Design review of the part built by this model. Coordinates are the model's own, in mm. Coordinates: 2 decimals unless noted, no trailing zeros. Write each loop counter-clockwise with the first axis right and the second up, starting at its lowest first coordinate (ties: lowest second). Pieces come first, ordered by that corner, then holes. Notation, with made-up numbers: (-28.5, 72.25) - (24.5, 72.25) arc R14 ccw to (24.5, 85.25) - close; hole circle Ø11 at (23.5, -20). An arc over 180 degrees is marked (long way). Answer as CSV lines item,"result". Start each with the question number.
Q1. Mouldability with a two-part tool opening along X and no side actions: class faces 1 (the face through (-73.454, -5, 16)), 2 (the face through (30.66, -4.93, -6.14)), 3 (the face through (-15, -5, -24.643)) as pulls with the +X half, pulls with the -X half, needs draft (parallel to the pull), parting line crosses it, or undercut.
Q2. We need section A-A (z = 32.5). Write out the cut boundary in (x, y), plus the area to 3 significant figures.
Q3. We need section B-B (y = -8). Write out the cut boundary in (x, z).
Q4. We need section C-C (x = -57). Write out the cut boundary in (y, z).
Q5. For line 1 along X through (y, z) = (-7, 35); line 2 along Z through (x, y) = (29, -3); line 3 along X through (y, z) = (-0.5, 31), list the stretches that pass through material, from the lowest coordinate up. Write a range as [from, to].
from build123d import *

# Parameters (mm, degrees)
F0_R     = 5
F1_DEPTH = 10


# Not quite as in the source:
# - the program builds the solid bodies; features that only make, move or delete a surface that nothing else refers to are left out


with BuildPart() as f1:
    # F0 (on Front) → F1 (new body)
    with BuildSketch(Plane.XZ):
        Polygon((45.889818927, 55.3569364734), (-73.4539608263, 55.3569364734), (-73.4539608263, 35.3569364734), (-73.4539608263, 5.3569364734), (45.889818927, 5.3569364734), (45.889818927, 35.3569364734), align=None)
        with BuildLine():
            ThreePointArc((-48.4539608263, 35.3569364734), (-53.4539608263, 30.3569364734), (-58.4539608263, 35.3569364734))
            ThreePointArc((-58.4539608263, 35.3569364734), (-53.4539608263, 40.3569364734), (-48.4539608263, 35.3569364734))
        make_face(mode=Mode.SUBTRACT)
        with Locations((25.889818927, 35.3569364734)):
            Circle(F0_R, mode=Mode.SUBTRACT)
        with BuildLine():
            Line((45.889818927, 5.3569364734), (-73.4539608263, 5.3569364734))
            Line((-73.4539608263, 5.3569364734), (-73.4539608263, -4.6430635266))
            Line((-73.4539608263, -4.6430635266), (20.889818927, -4.6430635266))
            ThreePointArc((20.889818927, -4.6430635266), (25.889818927, 0.3569364734), (30.889818927, -4.6430635266))
            Line((30.889818927, -4.6430635266), (45.889818927, -4.6430635266))
            Line((45.889818927, -4.6430635266), (45.889818927, 5.3569364734))
        make_face()
        with BuildLine():
            Line((20.889818927, -4.6430635266), (-73.4539608263, -4.6430635266))
            Line((-73.4539608263, -4.6430635266), (-73.4539608263, -24.6430635266))
            Line((-73.4539608263, -24.6430635266), (25.4732109606, -24.6430635266))
            Line((25.4732109606, -24.6430635266), (45.889818927, -24.6430635266))
            Line((45.889818927, -24.6430635266), (45.889818927, -4.6430635266))
            Line((45.889818927, -4.6430635266), (30.889818927, -4.6430635266))
            ThreePointArc((30.889818927, -4.6430635266), (25.889818927, -9.6430635266), (20.889818927, -4.6430635266))
        make_face()
    extrude(amount=F1_DEPTH)


solid = f1.part
Results list:
1,face 1,"pulls with the -X half"
1,face 2,"undercut"
1,face 3,"needs draft"
2,outline,"(-73.45, -10) - (-57.56, -10) - (-57.56, 0) - (-73.45, 0) - close; (-49.35, -10) - (21.79, -10) - (21.79, 0) - (-49.35, 0) - close; (29.99, -10) - (45.89, -10) - (45.89, 0) - (29.99, 0) - close"
2,area,"1,030 mm2"
3,outline,"(-73.45, -24.64) - (45.89, -24.64) - (45.89, 55.36) - (-73.45, 55.36) - close; hole circle Ø10 at (-53.45, 35.36); hole circle Ø10 at (25.89, -4.64); hole circle Ø10 at (25.89, 35.36)"
4,outline,"(-10, -24.64) - (0, -24.64) - (0, 31.83) - (-10, 31.83) - close; (-10, 38.88) - (0, 38.88) - (0, 55.36) - (-10, 55.36) - close"
5,line 1,"x = [-73.45, -58.44], [-48.47, 20.9], [30.88, 45.89]"
5,line 2,"z = [-24.64, -8.56], [-0.73, 31.44], [39.27, 55.36]"
5,line 3,"x = [-73.45, -55.91], [-51, 23.44], [28.34, 45.89]"
